Read the model definition and answer for the solid it produces. Units are mm, in the model's axes. Coordinates: 2 decimals unless noted, no trailing zeros. Write each loop counter-clockwise with the first axis right and the second up, starting at its lowest first coordinate (ties: lowest second). Pieces come first, ordered by that corner, then holes.
1) Each of these flat-tipped pins is pushed along its axis until it touches: pin 1 Ø0.9 at (y, z) = (6, -0.5) entering from -X; pin 2 Ø1.5 at (y, z) = (-18.5, 1) entering from +X; pin 3 Ø0.9 at (y, z) = (-7, 0.5) entering from -X. Where does it stop, or does it pass through?
2) The part is cut by section A-A (z = 0.1). Determine the outline of the cut face in (x, y), then the cut area to 3 significant figures.
3) The part is cut by section C-C (y = 6.5). Determine the outline of the cut face in (x, z).
4) The part is cut by section B-B (x = 4). Determine the outline of the cut face in (y, z).
5) The part is cut by section D-D (y = -27). Determine the outline of the cut face in (x, z), then the cut area to 3 significant figures.
6) Find the intervals of material crossed by line 1 (Y direction, x = -14, z = 1); line 2 (X direction, y = 15, z = 0.45); line 3 (Y direction, x = 7, z = 1.35), in increasing order.
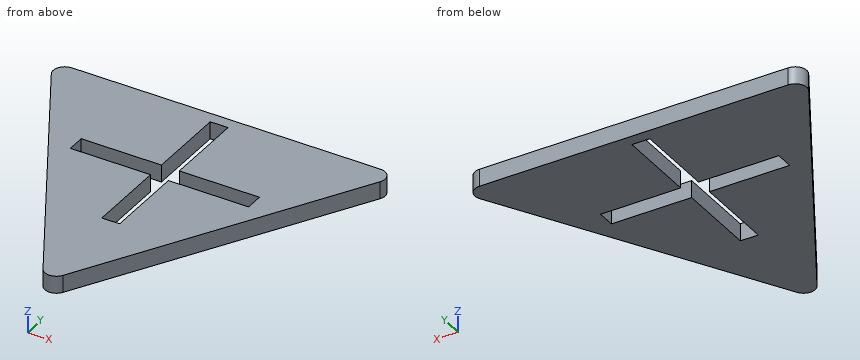
from build123d import *

# Parameters (mm, degrees)
BOSS_EXTRUDE1_DEPTH = 1.5


with BuildPart() as part:
    # Sketch1 → Boss-Extrude1 (new body, symmetric)
    with BuildSketch(Plane.XY):
        with BuildLine():
            ThreePointArc((28.578838325, 14.5), (28.578838325, 16.5), (26.846787517, 17.5))
            Line((26.846787517, 17.5), (-26.846787517, 17.5))
            ThreePointArc((-26.846787517, 17.5), (-28.578838325, 16.5), (-28.578838325, 14.5))
            Line((-28.578838325, 14.5), (-1.732050808, -32))
            ThreePointArc((-1.732050808, -32), (0, -33), (1.732050808, -32))
            Line((1.732050808, -32), (28.578838325, 14.5))
        make_face()
        Polygon((-1.55, 1.55), (-1.55, 15.5), (1.55, 15.5), (1.55, 1.55), (15.5, 1.55), (15.5, -1.55), (1.55, -1.55), (1.55, -15.5), (-1.55, -15.5), (-1.55, -1.55), (-15.5, -1.55), (-15.5, 1.55), align=None, mode=Mode.SUBTRACT)
    extrude(amount=BOSS_EXTRUDE1_DEPTH, both=True)


solid = part.part
Reported:
1. pin 1: stops at x = -23.93
1. pin 2: stops at x = 9.96
1. pin 3: stops at x = -16.43
2. outline: (-28.58, 14.5) - (-1.73, -32) arc R2 ccw to (1.73, -32) - (28.58, 14.5) arc R2 ccw to (26.85, 17.5) - (-26.85, 17.5) arc R2 ccw to start; hole (-15.5, -1.55) - (-1.55, -1.55) - (-1.55, -15.5) - (1.55, -15.5) - (1.55, -1.55) - (15.5, -1.55) - (15.5, 1.55) - (1.55, 1.55) - (1.55, 15.5) - (-1.55, 15.5) - (-1.55, 1.55) - (-15.5, 1.55) - close
2. area: 1,400 mm2
3. outline: (-23.96, -1.5) - (-1.55, -1.5) - (-1.55, 1.5) - (-23.96, 1.5) - close; (1.55, -1.5) - (23.96, -1.5) - (23.96, 1.5) - (1.55, 1.5) - close
4. outline: (-28.07, -1.5) - (-1.55, -1.5) - (-1.55, 1.5) - (-28.07, 1.5) - close; (1.55, -1.5) - (17.5, -1.5) - (17.5, 1.5) - (1.55, 1.5) - close
5. outline: (-4.62, -1.5) - (4.62, -1.5) - (4.62, 1.5) - (-4.62, 1.5) - close
5. area: 27.7 mm2
6. line 1: y = -10.75 to -1.55, 1.55 to 17.5
6. line 2: x = -28.78 to -1.55, 1.55 to 28.78
6. line 3: y = -22.88 to -1.55, 1.55 to 17.5
